from build123d import *

# Parameters (mm, degrees)
SKETCH1_W           = 29.5
SKETCH1_H           = 34
BOSS_EXTRUDE1_DEPTH = 13.5
SKETCH2_W           = 1.5
SKETCH2_H           = 3.8
SKETCH2_W_2         = 16.4
SKETCH2_H_2         = 3.5
CUT_EXTRUDE1_DEPTH  = 40.443789118


with BuildPart() as part:
    # Sketch1 → Boss-Extrude1 (new body)
    with BuildSketch(Plane.XY):
        Rectangle(SKETCH1_W, SKETCH1_H)
    extrude(amount=BOSS_EXTRUDE1_DEPTH)

    # Sketch2 → Cut-Extrude1 (cut, through all)
    with BuildSketch(Plane(origin=(0, 17, 0), x_dir=(1, 0, 0), z_dir=(0, 1, 0))):
        with Locations((-14, -1.9)):
            Rectangle(SKETCH2_W, SKETCH2_H)
        with Locations((0, -11.75)):
            Rectangle(SKETCH2_W_2, SKETCH2_H_2)
    cut_extrude1 = extrude(amount=-CUT_EXTRUDE1_DEPTH, mode=Mode.SUBTRACT)

    # Mirror1: Cut-Extrude1 across plane
    add(cut_extrude1.mirror(Plane(origin=(0, 0, 0), x_dir=(0, 0, 1), z_dir=(1, 0, 0))), mode=Mode.SUBTRACT)


solid = part.part
Build history of the part. All positions in model axes, mm. A direction names the side the tool comes from. Give positions to 0.01 mm unless a question says otherwise; leave off trailing zeros. Order: outer loops, then holes, each group sorted by start corner. A loop starts at its lowest first (then second) coordinate and runs counter-clockwise, first axis right, second up. Notation, with made-up numbers: M 36,80 L 47,80 A20 ccw 47,85 Z; hole C 21.5,25 d5. An arc over 180 degrees is marked long. Use one line per item in the form item = value.
1) Saw through at C-C (x = 0.75). Give the cut face in (y, z).
Calculated:
outline = M -17,0 L 17,0 L 17,10 L -17,10 Z
2) Saw through at D-D (z = 2). Give the cut face in (x, y).
Calculated:
outline = M -13.25,-17 L 13.25,-17 L 13.25,17 L -13.25,17 Z
3) Two-plate mould, pull along X, no slides. Class faces 1 (the face through (8.2, 0, 12)), 2 (the face through (-13.25, 0, 2)), 3 (the face through (14, 0, 3.8)): released by +X, released by -X, zero draft, split by the parting line, or undercut.
Calculated:
face_1 = undercut
face_2 = released by -X
face_3 = zero draft
4) Probe probe 1 along X at (y, z) = (-15, 12); probe 2 along Z at (x, y) = (-8, -12); probe 3 along X at (y, z) = (6, 3.25). List the from-to ranges inside material, lowest first.
Calculated:
probe_1 = -14.75 to -8.2, 8.2 to 14.75
probe_2 = 0 to 10
probe_3 = -13.25 to 13.25
5) Saw through at B-B (y = 3.5). Give the cut face in (x, z), plus the area to 3 significant figures.
Calculated:
outline = M -14.75,3.8 L -13.25,3.8 L -13.25,0 L 13.25,0 L 13.25,3.8 L 14.75,3.8 L 14.75,13.5 L 8.2,13.5 L 8.2,10 L -8.2,10 L -8.2,13.5 L -14.75,13.5 Z
area = 329 mm2
6) Drop flat-ended pins along their axis: pin 1 (13 mm diameter, centred on x = 1.5, y = 1.5, fed in from +Z); pin 2 (1.9 mm diameter, centred on y = 1, z = 2.5, fed in from -X); pin 3 (1.1 mm diameter, centred on y = -3, z = 2.5, fed in from +X). Give the stop position or say it passes through.
Calculated:
pin_1 = 10
pin_2 = -13.25
pin_3 = 13.25
7) Tool access for faces 4 (the face through (13.25, 0, 2)), 5 (the face through (0, 0, 10)), 6 (the face through (0, 17, 7)), 7 (the face through (-14, 0, 3.8)): list every direction of +Z, -Z, +X, -X, +Y, -Y with a clear straight run to the whole face (end or side of a thin tool).
Calculated:
face_4 = -Z, +X, +Y, -Y
face_5 = +Z, +Y, -Y
face_6 = +Z, -Z, +X, -X, +Y
face_7 = -Z, -X, +Y, -Y
8) Saw through at A-A (z = 11.25). Give the cut face in (x, y), plus the area to 3 significant figures.
Calculated:
outline = M -14.75,-17 L -8.2,-17 L -8.2,17 L -14.75,17 Z; M 8.2,-17 L 14.75,-17 L 14.75,17 L 8.2,17 Z
area = 445 mm2
